```python
from build123d import *

# Parameters (mm, degrees)
PAD_DEPTH = 575


with BuildPart() as part:
    # Sketch → Pad (new body)
    with BuildSketch(Plane.YZ):
        Polygon((0, 0), (35, 0), (35, 30), (0, 30), (0, 18), (6.5, 18), (6.5, 24.5), (28.5, 24.5), (28.5, 5.5), (6.5, 5.5), (6.5, 12), (0, 12), align=None)
    extrude(amount=PAD_DEPTH)


solid = part.part
```
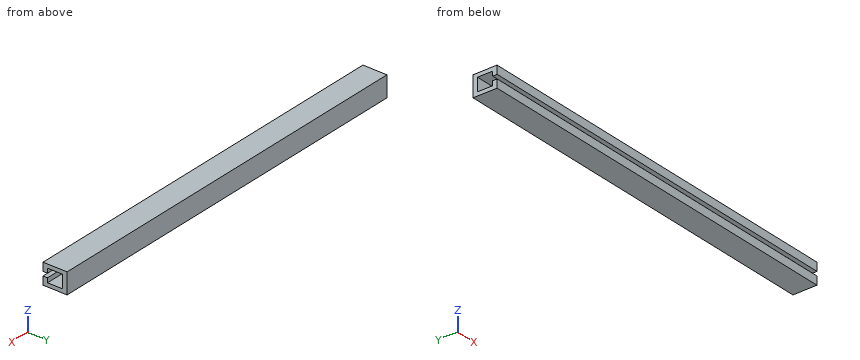
CAD build for the part. Positions are in the model's coordinates, mm. Coordinates: 2 decimals unless noted, no trailing zeros. Write each loop counter-clockwise with the first axis right and the second up, starting at its lowest first coordinate (ties: lowest second). Pieces come first, ordered by that corner, then holes. Notation, with made-up numbers: (-29, 17.25) -> (7, 17.25) arc R22 ccw to (7, 37.25) -> close; hole circle Ø9 at (64, 56.25). An arc over 180 degrees is marked (long way). Return JSON: item names as keys, results as strings. Group by question number.
Q1. Flat gauge pin, fed straight in: pin 1 (2 mm diameter, centred on x = 440, z = 13.5, fed in from -Y). Where does the tip first touch, or does it go through?
Q2. Drill centre lines: line 1 (Z direction, x = 486, y = 5.5); line 2 (Y direction, x = 90.5, z = 7.75); line 3 (Z direction, x = 385, y = 14). Where is each one in solid material? Low to high.
Q3. Cut at B-B, the plane x = 123. Give the cut face in (y, z), then the cut area to 3 significant figures.
Q4. Cut at A-A, the plane y = 18.5. Give the cut face in (x, z).
Returned:
{
 "1": {"pin 1": "stops at y = 28.5"},
 "2": {"line 1": "z = 0 to 12, 18 to 30", "line 2": "y = 0 to 6.5, 28.5 to 35", "line 3": "z = 0 to 5.5, 24.5 to 30"},
 "3": {"outline": "(0, 0) -> (35, 0) -> (35, 30) -> (0, 30) -> (0, 18) -> (6.5, 18) -> (6.5, 24.5) -> (28.5, 24.5) -> (28.5, 5.5) -> (6.5, 5.5) -> (6.5, 12) -> (0, 12) -> close", "area": "593 mm2"},
 "4": {"outline": "(0, 0) -> (575, 0) -> (575, 5.5) -> (0, 5.5) -> close; (0, 24.5) -> (575, 24.5) -> (575, 30) -> (0, 30) -> close"}
}
